from build123d import *

# Parameters (mm, degrees)
F0_W     = 25.4
F0_H     = 25.4
F1_DEPTH = 152.4
F3_D     = 17.4625
F3_DEPTH = 20.0025
F3_TIP   = 5.2462642799
F5_DEPTH = 304.801
F7_DEPTH = 304.801


with BuildPart() as f1:
    # F0 (on Right) → F1 (new body, symmetric)
    with BuildSketch(Plane.YZ):
        Rectangle(F0_W, F0_H)
    extrude(amount=F1_DEPTH, both=True)

    # F3
    with Locations(Plane.XY.offset(12.7)):
        with Locations((0, 0)):
            Hole(F3_D / 2, depth=F3_DEPTH)
            with Locations((0, 0, -(F3_DEPTH + F3_TIP / 2))):  # 118° drill point
                Cone(0, F3_D / 2, F3_TIP, mode=Mode.SUBTRACT)

    # F4 (on face) → F5 (cut, through all)
    with BuildSketch(Plane.YZ.offset(152.4)):
        Polygon((12.7, -12.7), (-12.7, 0), (-12.7, -12.7), align=None)
    extrude(amount=-F5_DEPTH, mode=Mode.SUBTRACT)

    # F6 (on face) → F7 (cut, through all)
    with BuildSketch(Plane.YZ.offset(152.4)):
        Polygon((12.2289045241, 12.7), (12.7, -8.89), (12.7, 12.7), align=None)
    extrude(amount=-F7_DEPTH, mode=Mode.SUBTRACT)


solid = f1.part
Here's how the part is built. I have some questions about the finished solid (model axes, mm). Coordinates: 2 decimals unless noted, no trailing zeros. Order: outer loops, then holes, each group sorted by start corner. A loop starts at its lowest first (then second) coordinate and runs counter-clockwise, first axis right, second up. Notation, with made-up numbers: (-23, 3) -> (30, 3) arc R18 ccw to (30, 19) -> close; hole circle Ø7 at (36, -16). An arc over 180 degrees is marked (long way). Answer in a Markdown table with one row per item.
(1) I want a section at D-D on x = 47. List the corners of the cut face in (y, z) for me.
Answer key:
| item | result |
|---|---|
| outline | (-12.7, 0) -> (12.7, -12.7) -> (12.7, -8.89) -> (12.23, 12.7) -> (-12.7, 12.7) -> close |
(2) I want a section at B-B on z = 7. List the corners of the cut face in (x, y) for me.
Answer key:
| item | result |
|---|---|
| outline | (-152.4, -12.7) -> (152.4, -12.7) -> (152.4, 12.35) -> (-152.4, 12.35) -> close; hole circle Ø17.46 at (0, 0) |
(3) I want a section at A-A on y = -3.75. List the corners of the cut face in (x, z) for me (3 decimals).
Answer key:
| item | result |
|---|---|
| outline | (-152.4, -4.475) -> (-7.885, -4.475) -> (-7.885, 12.7) -> (-152.4, 12.7) -> close; (7.885, -4.475) -> (152.4, -4.475) -> (152.4, 12.7) -> (7.885, 12.7) -> close |
(4) I want a section at C-C on x = 0. List the corners of the cut face in (y, z) for me.
Answer key:
| item | result |
|---|---|
| outline | (-12.7, 0) -> (-8.73, -1.98) -> (-8.73, 12.7) -> (-12.7, 12.7) -> close; (5.63, -9.17) -> (12.7, -12.7) -> (12.7, -8.89) -> (12.23, 12.7) -> (8.73, 12.7) -> (8.73, -7.3) -> close |
(5) Please list where these lines run through material, in increasing order: probe 1 along X at (y, z) = (0, -2.25); probe 2 along X at (y, z) = (2, 2.5); probe 3 along Y at (x, z) = (0, -1.75).
Answer key:
| item | result |
|---|---|
| probe 1 | -152.4 to -8.73, 8.73 to 152.4 |
| probe 2 | -152.4 to -8.5, 8.5 to 152.4 |
| probe 3 | -9.2 to -8.73, 8.73 to 12.54 |
(6) Thinking about a two-plate mould opening in Y: for faces 1 (the face through (152.4, 0, 3)), 2 (the face through (1.137, 8.657, 2.559)), 3 (the face through (2, -12.7, 6)), which applies, +Y half, -Y half, draft (parallel to the pull), parting line (faces both ways), or undercut?
Answer key:
| item | result |
|---|---|
| face 1 | draft |
| face 2 | undercut |
| face 3 | -Y half |
(7) Will these pins go through, and if not, where does the flat tip stop? pin 1 Ø4 at (x, z) = (48, -4.5) entering from +Y; pin 2 Ø5 at (x, z) = (-1, -3.5) entering from -Y.
Answer key:
| item | result |
|---|---|
| pin 1 | y = 12.65 |
| pin 2 | y = -10.7 |
